Part model, mm, in its own coordinate system. A direction names the side the tool comes from. Round coordinates to 2 decimals unless told otherwise and drop trailing zeros. Write each loop counter-clockwise with the first axis right and the second up, starting at its lowest first coordinate (ties: lowest second). Pieces come first, ordered by that corner, then holes. Notation, with made-up numbers: M 24,85 L 69,85 A30 cw 69,110 Z; hole C 81.5,3 d11. An arc over 180 degrees is marked long. One line per question, with ' | ' between items. Start each with the question number.
1) Wall check: probe 1 along Z at (x, y) = (79.5, 22); probe 2 along X at (y, z) = (39.5, 14). Give the ranges that are in metal, low to high. Write a range as [from, to].
2) Saw through at C-C (y = 24.5). List the corners of the cut face in (x, z), plus the area to 3 significant figures.
3) Tool access for faces 5 (the face through (50, 35, 10)), 6 (the face through (136.71, 9.86, 53.3)), 7 (the face through (101, 42, 20)): list every direction of +Z, -Z, +X, -X, +Y, -Y with a clear straight run to the whole face (end or side of a thin tool).
4) Mould opens along X. For faces 1 (the face through (76, 20, 38)), 2 (the face through (80.175, 54.153, 9.86)), 3 (the face through (15.75, 9.86, 8.67)), 4 (the face through (65.09, 9.86, 55.28)) say: pulls with the +X half, pulls with the -X half, needs draft (parallel to the pull), parting line crosses it, or undercut.
5) Saw through at A-A (y = 57.5). List the corners of the cut face in (x, z).
6) Saw through at D-D (x = 90). List the corners of the cut face in (y, z), plus the area to 3 significant figures.
7) Saw through at B-B (x = 14.5). List the corners of the cut face in (y, z), plus the area to 3 significant figures.
8) Drop flat-ended pins along their axis: pin 1 Ø1 at (x, y) = (50, 24) entering from +Z; pin 2 Ø4 at (x, z) = (47, 33.5) entering from -Y; pin 3 Ø10 at (y, z) = (41.5, 11.5) entering from -X. Give the stop position or say it passes through.
```python
from build123d import *

# Parameters (mm, degrees)
BOSS_EXTRUDE1_DEPTH    = 20
BOSS_EXTRUDE4_DEPTH    = 20
FILLET1_R              = 25
FILLET2_R              = 12
F_20_0MM_DOWEL_HOLE2_D = 20
F_20_0MM_DOWEL_HOLE4_D = 20
F_20_0MM_DOWEL_HOLE5_D = 20


with BuildPart() as part:
    # Sketch1 → Boss-Extrude1 (new body)
    with BuildSketch(Plane(origin=(0, 0, 0), x_dir=(1, 0, 0), z_dir=(0, 1, 0))):
        with BuildLine():
            Line((0, 0), (150, 0))
            Line((150, 0), (150, -51.689934114))
            ThreePointArc((150, -51.689934114), (139.12642407, -72.316231479), (115.964468561, -75))
            Line((115.964468561, -75), (12.771574849, -35))
            ThreePointArc((12.771574849, -35), (3.498962108, -27.653086547), (0, -16.351947291))
            Line((0, -16.351947291), (0, 0))
        make_face()
    extrude(amount=BOSS_EXTRUDE1_DEPTH)

    # Sketch3 → Boss-Extrude4 (add)
    with BuildSketch(Plane.XY):
        Polygon((150, 0), (50, 0), (50, 80), (150, 60), align=None)
    extrude(amount=BOSS_EXTRUDE4_DEPTH)

    # Fillet1
    fillet1_edges = [part.edges().sort_by_distance(p)[0] for p in [
        (50, 80, 10),
    ]]
    fillet(fillet1_edges, radius=FILLET1_R)

    # Fillet2
    fillet2_edges = [part.edges().sort_by_distance(p)[0] for p in [
        (150, 60, 10),
    ]]
    fillet(fillet2_edges, radius=FILLET2_R)

    # Ø20.0mm Dowel Hole2 (through all)
    with Locations(Plane.XY.offset(20)):
        with Locations((70.185160084, 53.713740801)):
            Hole(F_20_0MM_DOWEL_HOLE2_D / 2)

    # Ø20.0mm Dowel Hole4 (through all)
    with Locations(Plane(origin=(0, 20, 0), x_dir=(1, 0, 0), z_dir=(0, 1, 0))):
        with Locations((21.126269386, -17.1033247)):
            Hole(F_20_0MM_DOWEL_HOLE4_D / 2)

    # Ø20.0mm Dowel Hole5 (through all)
    with Locations(Plane(origin=(0, 20, 0), x_dir=(1, 0, 0), z_dir=(0, 1, 0))):
        with Locations((126.71878139, -53.737461518)):
            Hole(F_20_0MM_DOWEL_HOLE5_D / 2)


solid = part.part
```
Answer key:
1) probe 1: z = [0, 20] | probe 2: x = [50, 150]
2) outline: M 50,0 L 150,0 L 150,20 L 50,20 Z | area: 2,000 mm2
3) face 5: +Z, -Z, -X, +Y | face 6: +Y, -Y | face 7: +Z, +X, -X, +Y
4) face 1: needs draft | face 2: undercut | face 3: undercut | face 4: pulls with the -X half
5) outline: M 51.31,0 L 60.93,0 L 60.93,20 L 51.31,20 Z; M 79.44,0 L 147.5,0 L 147.5,20 L 79.44,20 Z
6) outline: M 0,0 L 72,0 L 72,20 L 20,20 L 20,64.94 L 0,64.94 Z | area: 2,340 mm2
7) outline: M 0,0 L 20,0 L 20,9.61 L 0,9.61 Z; M 0,24.59 L 20,24.59 L 20,35.67 L 0,35.67 Z | area: 414 mm2
8) pin 1: stops at z = 20 | pin 2: stops at y = 0 | pin 3: stops at x = 50
